For this review, take the finished solid that the model builds, in its own axes (mm). Face numbers are marked on the shaded views. Give positions to 0.01 mm unless a question says otherwise; leave off trailing zeros. Loops run counter-clockwise (first coordinate to the right, second up) from the corner with the lowest first, then second, coordinate; pieces in that order, holes last. Notation, with made-up numbers: (40.5, -19) - (91.5, -19) arc R28 cw to (91.5, 11) - close; hole circle Ø11 at (-22.5, 53.25). An arc over 180 degrees is marked (long way). Use CSV: the item, a comma, the result in double quotes. Start each with the question number.
1. For pin 1 (17.5 mm diameter, centred on x = 0, z = 0, fed in from -Y), flat-tipped, find the tip position at first contact; note if it passes through.
2. Take a section at B-B on z = 0. Give the boundary of the cut face in (x, y), plus the area to 3 significant figures.
3. Take a section at C-C on y = 10. Give the boundary of the cut face in (x, z), plus the area to 3 significant figures.
4. Mouldability with a two-part tool opening along Z and no side actions: class the marked faces 1, 2 and 3 as pulls with the +Z half, pulls with the -Z half, needs draft (parallel to the pull), parting line crosses it, or undercut.
5. Wall thickness on line 1 (Z direction, x = 0, y = 22); line 2 (Z direction, x = 23, y = -35.5); line 3 (Z direction, x = -3, y = -28): over which ranges is each line inside the solid? List them lowest first.
6. Take a section at A-A on x = 0. Give the boundary of the cut face in (y, z).
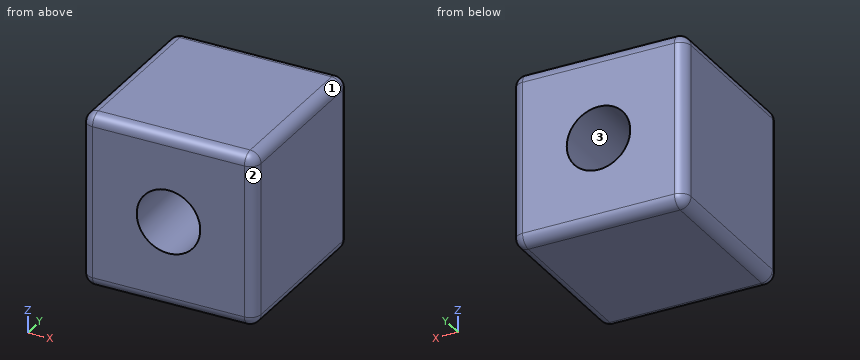
```python
from build123d import *

# Parameters (mm, degrees)
F0_W     = 80
F0_H     = 80
F1_DEPTH = 40
F2_R     = 5
F3_R     = 14.637142
F4_DEPTH = 80.001


with BuildPart() as f1:
    # F0 (on Top) → F1 (new body, symmetric)
    with BuildSketch(Plane.XY):
        Rectangle(F0_W, F0_H)
    extrude(amount=F1_DEPTH, both=True)

    # F2
    f2_edges = [f1.edges().sort_by_distance(p)[0] for p in [
        (40, -40, 0),
        (0, -40, -40),
        (-40, -40, 0),
        (-40, 0, -40),
        (40, 0, -40),
        (0, 40, -40),
        (-40, 40, 0),
        (-40, 0, 40),
        (0, -40, 40),
        (0, 40, 40),
        (40, 0, 40),
        (40, 40, 0),
    ]]
    fillet(f2_edges, radius=F2_R)

    # F3 (on face) → F4 (cut, through all)
    with BuildSketch(Plane.XZ.offset(40)):
        Circle(F3_R)
    extrude(amount=-F4_DEPTH, mode=Mode.SUBTRACT)


solid = f1.part
```
Check result:
1,pin 1,"passes through"
2,outline,"(-40, -35) arc R5 ccw to (-35, -40) - (-14.64, -40) - (-14.64, 40) - (-35, 40) arc R5 ccw to (-40, 35) - close; (14.64, -40) - (35, -40) arc R5 ccw to (40, -35) - (40, 35) arc R5 ccw to (35, 40) - (14.64, 40) - close"
2,area,"4,040 mm²"
3,outline,"(-40, -35) arc R5 ccw to (-35, -40) - (35, -40) arc R5 ccw to (40, -35) - (40, 35) arc R5 ccw to (35, 40) - (-35, 40) arc R5 ccw to (-40, 35) - close; hole circle Ø29.27 at (0, 0)"
3,area,"5,710 mm²"
4,face 1,"pulls with the +Z half"
4,face 2,"needs draft"
4,face 3,"undercut"
5,line 1,"z = -40 to -14.64, 14.64 to 40"
5,line 2,"z = -39.97 to 39.97"
5,line 3,"z = -40 to -14.33, 14.33 to 40"
6,outline,"(-40, -35) arc R5 ccw to (-35, -40) - (35, -40) arc R5 ccw to (40, -35) - (40, -14.64) - (-40, -14.64) - close; (-40, 14.64) - (40, 14.64) - (40, 35) arc R5 ccw to (35, 40) - (-35, 40) arc R5 ccw to (-40, 35) - close"
